```python
from build123d import *

# Parameters (mm, degrees)
SKETCH_1_W      = 7.6
SKETCH_1_H      = 1.9
EXTRUDE_1_DEPTH = 2


with BuildPart() as part:
    # 草图1 → 凸台-拉伸1 (new body)
    with BuildSketch(Plane(origin=(0, 0, 0), x_dir=(1, 0, 0), z_dir=(0, 1, 0))):
        Polygon((0, 33.8), (0, 0), (5, 0), (5, -2), (12.6, -2), (12.6, 0), (16.6, 0), (16.6, 1), (17.6, 1), (17.6, 33.8), (16.6, 33.8), (16.6, 34.8), (12.6, 34.8), (12.6, 36.8), (5, 36.8), (5, 34.8), (1, 34.8), (1, 33.8), align=None)
        with Locations((8.8, 17.95)):
            Rectangle(SKETCH_1_W, SKETCH_1_H, mode=Mode.SUBTRACT)
    extrude(amount=EXTRUDE_1_DEPTH)


solid = part.part
```
Model file for the job. Use its own axes, mm. A direction names the side the tool comes from. Round coordinates to 2 decimals unless told otherwise and drop trailing zeros. Write each loop counter-clockwise with the first axis right and the second up, starting at its lowest first coordinate (ties: lowest second). Pieces come first, ordered by that corner, then holes. Notation, with made-up numbers: M -27.75,-2 L -7.75,-2 A16 cw -7.75,8 Z; hole C 87,-4 d1. An arc over 180 degrees is marked long. Put each result on its own line as item: value.
Item 1: Cut at A-A (x = 8). List the corners of the cut face in (y, z).
Responses:
outline: M 0,-36.8 L 2,-36.8 L 2,-18.9 L 0,-18.9 Z; M 0,-17 L 2,-17 L 2,2 L 0,2 Z
Item 2: Mould opens along Z. For faces 1 (the flat face through (17.6, 1, -17)), 2 (the flat face through (15, 1, 0)), 3 (the flat face through (12.6, 1, -18)), 4 (the flat face through (9, 1, -17)) say: +Z half, -Z half, draft (parallel to the pull), parting line (faces both ways), or undercut.
Responses:
face 1: draft
face 2: +Z half
face 3: undercut
face 4: undercut
Item 3: Tool access for faces 5 (the flat face through (9, 1, -18.9)), 6 (the flat face through (15, 1, -34.8)), 7 (the flat face through (12.6, 1, 1)), 8 (the flat face through (2, 1, 0)), 9 (the flat face through (3, 1, -34.8)): list every direction of +Z, -Z, +X, -X, +Y, -Y with a clear straight run to the whole face (end or side of a thin tool).
Responses:
face 5: +Y, -Y
face 6: -Z, +X, +Y, -Y
face 7: +Z, +X, +Y, -Y
face 8: +Z, -X, +Y, -Y
face 9: -Z, -X, +Y, -Y
Item 4: Cut at B-B (y = 1.1). List the corners of the cut face in (x, z).
Responses:
outline: M 0,-33.8 L 1,-33.8 L 1,-34.8 L 5,-34.8 L 5,-36.8 L 12.6,-36.8 L 12.6,-34.8 L 16.6,-34.8 L 16.6,-33.8 L 17.6,-33.8 L 17.6,-1 L 16.6,-1 L 16.6,0 L 12.6,0 L 12.6,2 L 5,2 L 5,0 L 0,0 Z; hole M 5,-18.9 L 12.6,-18.9 L 12.6,-17 L 5,-17 Z
Item 5: Cut at C-C (x = 14.5). List the corners of the cut face in (y, z).
Responses:
outline: M 0,-34.8 L 2,-34.8 L 2,0 L 0,0 Z
Item 6: Probe L1, parallel to Z at x = 6.5, y = 1.4; L2, parallel to Z at x = 14.25, y = 1.4. List the from-to ranges inside material, lowest first. Write a range as from..to.
Responses:
L1: -36.8..-18.9, -17..2
L2: -34.8..0
Item 7: Flat gauge pins, fed straight in: P1, Ø1.1, axis at x = 0.5, y = 0.5, coming from the -Z side; P2, Ø1.1, axis at x = 17.5, y = 1, coming from the +Z side; P3, Ø0.8, axis at y = 1.5, z = -34.5, coming from the +X side. Where does each tip first touch, or does it go through?
Responses:
P1: z = -34.8
P2: z = -1
P3: x = 16.6
